Read the model definition and answer for the solid it produces. Units are mm, in the model's axes. A direction names the side the tool comes from. Round coordinates to 2 decimals unless told otherwise and drop trailing zeros. Write each loop counter-clockwise with the first axis right and the second up, starting at its lowest first coordinate (ties: lowest second). Pieces come first, ordered by that corner, then holes.
from build123d import *

# Parameters (mm, degrees)
F0_R     = 3.1652149855
F1_DEPTH = 7
F3_DEPTH = 25
F5_DEPTH = 3
F7_R     = 3.1652149855
F7_R_2   = 1.7
F8_DEPTH = 2


with BuildPart() as f1:
    # F0 (on Top) → F1 (new body)
    with BuildSketch(Plane.XY):
        with BuildLine():
            Line((7.6635631778, -0.8648966905), (21.4957091957, 46.0475608706))
            ThreePointArc((21.4957091957, 46.0475608706), (0, 67.5432700664), (-21.4957091957, 46.0475608706))
            Line((-21.4957091957, 46.0475608706), (-7.6635631778, -0.8648966905))
            Line((-7.6635631778, -0.8648966905), (7.6635631778, -0.8648966905))
        make_face()
        with BuildLine():
            ThreePointArc((17, 49.0475608706), (20, 46.0475608706), (17, 43.0475608706))
            Line((17, 43.0475608706), (5.6355242597, 40.232100229))
            Line((5.6355242597, 40.232100229), (3, 29.0475608706))
            ThreePointArc((3, 29.0475608706), (0, 26.0475608706), (-3, 29.0475608706))
            Line((-3, 29.0475608706), (-5.6355242597, 40.232100229))
            Line((-5.6355242597, 40.232100229), (-17, 43.0475608706))
            ThreePointArc((-17, 43.0475608706), (-20, 46.0475608706), (-17, 49.0475608706))
            Line((-17, 49.0475608706), (-5.6355242597, 51.8630215122))
            Line((-5.6355242597, 51.8630215122), (-3, 63.0475608706))
            ThreePointArc((-3, 63.0475608706), (0, 66.0475608706), (3, 63.0475608706))
            Line((3, 63.0475608706), (5.6355242597, 51.8630215122))
            Line((5.6355242597, 51.8630215122), (17, 49.0475608706))
        make_face(mode=Mode.SUBTRACT)
        with BuildLine():
            Line((5.6355242597, 40.232100229), (17, 43.0475608706))
            ThreePointArc((17, 43.0475608706), (20, 46.0475608706), (17, 49.0475608706))
            Line((17, 49.0475608706), (5.6355242597, 51.8630215122))
            Line((5.6355242597, 51.8630215122), (3, 63.0475608706))
            ThreePointArc((3, 63.0475608706), (0, 66.0475608706), (-3, 63.0475608706))
            Line((-3, 63.0475608706), (-5.6355242597, 51.8630215122))
            Line((-5.6355242597, 51.8630215122), (-17, 49.0475608706))
            ThreePointArc((-17, 49.0475608706), (-20, 46.0475608706), (-17, 43.0475608706))
            Line((-17, 43.0475608706), (-5.6355242597, 40.232100229))
            Line((-5.6355242597, 40.232100229), (-3, 29.0475608706))
            ThreePointArc((-3, 29.0475608706), (0, 26.0475608706), (3, 29.0475608706))
            Line((3, 29.0475608706), (5.6355242597, 40.232100229))
        make_face()
        with Locations((0, 46.0475608706)):
            Circle(F0_R, mode=Mode.SUBTRACT)
    extrude(amount=F1_DEPTH)

    # F2 (on Right) → F3 (join)
    with BuildSketch(Plane.YZ):
        with BuildLine():
            Line((-22.1495963633, 4.7701704316), (9.0307667851, 4.7701704316))
            ThreePointArc((9.0307667851, 4.7701704316), (9.0416852427, 4.809647179), (9.0525037393, 4.8491514374))
            ThreePointArc((9.0525037393, 4.8491514374), (-6.5885383667, 20.6088531813), (-22.1495963633, 4.7701704316))
        make_face()
        Polygon((9.0307667851, 4.168368876), (9.0307667851, 4.7701704316), (-22.1495963633, 4.7701704316), (-22.1495963633, 0), (9.0307667851, 0), align=None)
        with BuildLine():
            ThreePointArc((9.0525037393, 4.8491514374), (9.0416852427, 4.809647179), (9.0307667851, 4.7701704316))
            Line((9.0307667851, 4.7701704316), (9.0307667851, 4.168368876))
            ThreePointArc((9.0307667851, 4.168368876), (9.0453507005, 4.5086415251), (9.0525037393, 4.8491514374))
        make_face()
    extrude(amount=F3_DEPTH)

    # F4: F1 across plane


with BuildPart() as f1_1:
    add(f1.part)
    add(f1.part.mirror(Plane.YZ))

    # F0 (on Top) → F5 (cut)
    with BuildSketch(Plane.XY):
        with BuildLine():
            Line((5.6355242597, 40.232100229), (17, 43.0475608706))
            ThreePointArc((17, 43.0475608706), (20, 46.0475608706), (17, 49.0475608706))
            Line((17, 49.0475608706), (5.6355242597, 51.8630215122))
            Line((5.6355242597, 51.8630215122), (3, 63.0475608706))
            ThreePointArc((3, 63.0475608706), (0, 66.0475608706), (-3, 63.0475608706))
            Line((-3, 63.0475608706), (-5.6355242597, 51.8630215122))
            Line((-5.6355242597, 51.8630215122), (-17, 49.0475608706))
            ThreePointArc((-17, 49.0475608706), (-20, 46.0475608706), (-17, 43.0475608706))
            Line((-17, 43.0475608706), (-5.6355242597, 40.232100229))
            Line((-5.6355242597, 40.232100229), (-3, 29.0475608706))
            ThreePointArc((-3, 29.0475608706), (0, 26.0475608706), (3, 29.0475608706))
            Line((3, 29.0475608706), (5.6355242597, 40.232100229))
        make_face()
        with Locations((0, 46.0475608706)):
            Circle(F0_R, mode=Mode.SUBTRACT)
    extrude(amount=F5_DEPTH, mode=Mode.SUBTRACT)

    # F7 (on offset) → F8 (join)
    with BuildSketch(Plane.XY.offset(3.556)):
        with Locations((0, 46.0307821631)):
            Circle(F7_R)
        with Locations((0, 46.0307821631)):
            Circle(F7_R_2, mode=Mode.SUBTRACT)
    extrude(amount=F8_DEPTH)


solid = f1_1.part
Q1. Determine the mould class of faces 4 (the cylindrical face through (-0.412, 49.186, 5.861)), 5 (the flat face through (0, 39, 7)), 6 (the flat face through (15.946, 27.227, 3.451)), 7 (the flat face through (3, 48, 3)) for opening direction Z: pulls with the +Z half, pulls with the -Z half, needs draft (parallel to the pull), parting line crosses it, or undercut.
Verdict:
face 4: undercut
face 5: pulls with the +Z half
face 6: needs draft
face 7: pulls with the -Z half
Q2. Section A-A (x = 7) is taken. Determine the outline of the cut face in (y, z), then the cut area to 3 significant figures.
Verdict:
outline: (-22.15, 0) - (40.57, 0) - (40.57, 3) - (51.52, 3) - (51.52, 0) - (66.37, 0) - (66.37, 7) - (8.93, 7) arc R15.6 ccw to (-22.15, 4.77) - close
area: 907 mm2
Q3. Flat-ended cylindrical pins translate along their axes: pin 1 Ø6 at (x, z) = (16, 4) entering from +Y; pin 2 Ø2.5 at (x, y) = (0, 46.03) entering from +Z; pin 3 Ø4.5 at (x, z) = (-19, 1) entering from +Y; pin 4 Ø2 at (x, z) = (17.5, 3) entering from +Y. Find the tip coordinate at first contact, or state that the pin passes through.
Verdict:
pin 1: stops at y = 63.17
pin 2: passes through
pin 3: stops at y = 59.52
pin 4: stops at y = 59.82
Q4. Section C-C (z = 14.75) is taken. Determine the outline of the cut face in (x, y).
Verdict:
outline: (-25, -18.74) - (25, -18.74) - (25, 5.64) - (-25, 5.64) - close
Q5. Section D-D (x = -7.5) is taken. Determine the outline of the cut face in (y, z).
Verdict:
outline: (-22.15, 0) - (40.69, 0) - (40.69, 3) - (51.4, 3) - (51.4, 0) - (66.19, 0) - (66.19, 7) - (8.93, 7) arc R15.6 ccw to (-22.15, 4.77) - close
Q6. Straight lines are drawn through the part: probe 1 along Z at (x, y) = (-2.5, 57.5); probe 2 along Z at (x, y) = (15.5, 58); probe 3 along X at (y, z) = (22.5, 6). For each, find the intervals that lie inside material, in ascending order.
Verdict:
probe 1: z = 3 to 7
probe 2: z = 0 to 7
probe 3: x = -14.55 to 14.55
Q7. Section B-B (y = 31.5) is taken. Determine the outline of the cut face in (x, z).
Verdict:
outline: (-17.21, 0) - (-3.58, 0) - (-3.58, 3) - (3.58, 3) - (3.58, 0) - (17.21, 0) - (17.21, 7) - (-17.21, 7) - close
Q8. Which of the six approach directions +Z, -Z, +X, -X, +Y, -Y give full straight-line access (tool end or side, diameter ignored) to faces 1 (the flat face through (0, -22.15, 2)), 2 (the cylindrical face through (0.066, 66.047, 1.479)), 3 (the flat face through (-25, -7, 8))?
Verdict:
face 1: +Z, -Z, +X, -X, -Y
face 2: -Z
face 3: +Z, -Z, -X, +Y, -Y
